Work out the finished part from the listing and answer in its coordinate system (mm). A direction names the side the tool comes from. Give positions to 0.01 mm unless a question says otherwise; leave off trailing zeros. Order: outer loops, then holes, each group sorted by start corner. A loop starts at its lowest first (then second) coordinate and runs counter-clockwise, first axis right, second up.
Autodesk Inventor part; units mm, degrees
ref_plane "YZ Plane" through (0, 0, 0) normal (1, 0, 0) x (0, 1, 0)
ref_plane "XZ Plane" through (0, 0, 0) normal (0, 1, 0) x (-1, 0, 0)
ref_plane "XY Plane" through (0, 0, 0) normal (0, 0, 1) x (1, 0, 0)
sketch "Sketch1" plane through (0, 0, 0) normal (0, 0, 1) x (1, 0, 0)
  line L0 (0, 0) -> (-25.4, 0)
  line L1 (-25.4, 0) -> (-25.4, 25.4)
  line L2 (-25.4, 25.4) -> (0, 25.4)
  line L3 (0, 25.4) -> (0, 0)
  line L4 (-3.175, 22.225) -> (-22.225, 22.225)
  line L5 (-22.225, 22.225) -> (-22.225, 3.175)
  line L6 (-22.225, 3.175) -> (-3.175, 3.175)
  line L7 (-3.175, 3.175) -> (-3.175, 22.225)
  dimension "d2" = 25.4
  dimension "d4" = 25.4
  dimension "d5" = 3.175
extrude "Extrusion1" add sketch "Sketch1" along normal blind 72.39
sketch "Sketch2" plane through (-25.4, 25.4, 0) normal (0, 1, 0) x (1, 0, 0)
  line L0 (0, 0) -> (25.4, 0)
  line L1 (0, 0) -> (0, -72.39)
  line L2 (0, 0) -> (0, -1.905)
  line L3 (12.7, 0) -> (12.7, -1.905)
  line L4 (12.7, -1.905) -> (0, 0)
  line L5 (12.7, -1.905) -> (25.4, 0)
  line L6 (25.4, 0) -> (25.4, -72.39)
  line L7 (12.7, -1.905) -> (8.9322, -27.024)
  line L8 (12.7, -1.905) -> (16.4678, -27.024)
  line L9 (0, -25.6842) -> (8.9322, -27.024)
  line L10 (16.4678, -27.024) -> (25.4, -25.6842)
  line L11 (8.9322, -27.024) -> (17.0812, -28.2463)
  line L12 (16.4678, -27.024) -> (8.6718, -28.1934)
  dimension "d8" = 1.905
  dimension "d9" = 1.905
  dimension "d23" = 25.4
  dimension "d24" = 90
  dimension "d25" = 25.4
  dimension "d26" = 90
extrude "Extrusion2" cut sketch "Sketch2" against normal blind 25.4 contours L4 L7 L9 L1 | L0 L3 L4 | L0 L5 L3 | L5 L6 L10 L8
sketch "Sketch3" plane through (-25.4, 25.4, 72.39) normal (0, 1, 0) x (1, 0, 0)
  line L0 (25.4, 0) -> (0, 0)
  line L1 (25.4, 46.7058) -> (25.4, 0)
  line L2 (12.7, 0) -> (12.7, 70.485) construction
  line L3 (12.7, 0) -> (12.7, 6.35)
  circle A0 centre (12.7, 6.35) radius 3.3782
  circle A1 centre (12.7, 19.05) radius 3.3782
  circle A2 centre (12.7, 31.75) radius 3.3782
  point P0 (25.4, 72.39)
  dimension "d12" = 6.35
  dimension "d13" = 6.7564
  dimension "d16" = 12.7
extrude "Extrusion3" cut sketch "Sketch3" against normal blind 25.4
sketch "Sketch4" plane through (-12.7, 0, 15.24) normal (0, -1, 0) x (1, 0, 0)
  arc A0 (-1.55, -3.0016) -> (1.55, -3.0016) centre (0, 0) ccw
  line L0 (-3.7678, 11.784) -> (0, -13.335)
  line L1 (0, -13.335) -> (3.7678, 11.784)
  point P0 (12.7, -15.24)
extrude "Extrusion4" cut sketch "Sketch4" against normal blind 25.4
sketch "Sketch5" plane through (-25.4, 0, 72.39) normal (0, -1, 0) x (1, 0, 0)
  arc A0 (15.0625, -54.7353) -> (10.3375, -54.7353) centre (12.7, -57.15) ccw
  line L0 (12.7, -70.485) -> (16.4678, -45.366)
  line L1 (8.9322, -45.366) -> (12.7, -70.485)
  circle A1 centre (12.7, -44.45) radius 3.3782
  line L2 (8.9322, -45.366) -> (12.7, -44.45)
  line L3 (12.7, -44.45) -> (16.4678, -45.366)
  point P0 (25.4, -72.39)
extrude "Extrusion5" cut sketch "Sketch5" against normal blind 25.4 contours A0 L1 L2 A1 L3 L0 | A1 L2 L3 picked at (14.5428, -45.7157)
sketch "Sketch8" plane through (-12.7, 25.4, 15.24) normal (0, 1, 0) x (1, 0, 0)
  arc A0 (-2.3625, -2.4147) -> (2.3625, -2.4147) centre (0, 0) ccw
  line L0 (2.3625, -2.4147) -> (1.55, 3.0016)
  arc A1 (1.55, 3.0016) -> (-1.55, 3.0016) centre (0, 0) ccw
  line L1 (-1.55, 3.0016) -> (-2.3625, -2.4147)
  point P0 (12.7, 15.24)
extrude "Extrusion6" cut sketch "Sketch8" against normal blind 25.4
properties part number "V mount" material "Aluminum 6061"
1. The part is cut by section C-C (z = 35.5). Write down the section's boundary in (x, y) (3 decimals), then the cut area to 3 significant figures.
Findings below:
outline: (-25.4, 0) - (0, 0) - (0, 25.4) - (-25.4, 25.4) - close; hole (-22.225, 3.175) - (-3.175, 3.175) - (-3.175, 22.225) - (-22.225, 22.225) - close
area: 282 mm2
2. A straight line is drawn through the part: probe 1 along Y at (x, z) = (-21.75, 45.5) (3 decimals). Find the intervals that lie inside material, in ascending order.
Findings below:
probe 1: y = 0 to 3.175, 22.225 to 25.4
3. The part is cut by section A-A (z = 66.04). Write down the section's boundary in (x, y) (3 decimals), then the cut area to 3 significant figures.
Findings below:
outline: (-25.4, 0) - (-16.078, 0) - (-16.078, 3.175) - (-22.225, 3.175) - (-22.225, 22.225) - (-16.078, 22.225) - (-16.078, 25.4) - (-25.4, 25.4) - close; (-9.322, 0) - (0, 0) - (0, 25.4) - (-9.322, 25.4) - (-9.322, 22.225) - (-3.175, 22.225) - (-3.175, 3.175) - (-9.322, 3.175) - close
area: 239 mm2
4. The part is cut by section D-D (y = 12.75). Write down the section's boundary in (x, z) (3 decimals).
Findings below:
outline: (-25.4, 25.684) - (-22.225, 26.16) - (-22.225, 72.39) - (-25.4, 72.39) - close; (-3.175, 26.16) - (0, 25.684) - (0, 72.39) - (-3.175, 72.39) - close
5. Which of the six approach directions +Z, -Z, +X, -X, +Y, -Y give full straight-line access (tool end or side, diameter ignored) to faces 4 (the face through (-2, 13, 72.39)), 5 (the face through (-22.981, 12.878, 26.047)), 6 (the face through (-22.225, 13, 49))?
Findings below:
face 4: +Z, +X, -X, +Y, -Y
face 5: -Z, +Y, -Y
face 6: +Z, -Z
6. The part is cut by section B-B (y = 23). Write down the section's boundary in (x, z).
Findings below:
outline: (-25.4, 25.68) - (-16.47, 27.02) - (-12.7, 27.94) - (-8.93, 27.02) - (0, 25.68) - (0, 72.39) - (-25.4, 72.39) - close; hole circle Ø6.76 at (-12.7, 40.64); hole circle Ø6.76 at (-12.7, 53.34); hole circle Ø6.76 at (-12.7, 66.04)
7. The mould has two halves that part along Z. Classify faces 1 (the face through (-3.175, 13, 49)), 2 (the face through (-13.43, 1.61, 56.64)), 3 (the face through (-14.61, 23.79, 27.476)): pulls with the +Z half, pulls with the -Z half, needs draft (parallel to the pull), parting line crosses it, or undercut.
Findings below:
face 1: needs draft
face 2: undercut
face 3: pulls with the -Z half
8. Given P1, Ø6, axis at x = -12.7, z = 53.34, coming from the -Y side; P2, Ø4, axis at x = -10, y = 4.5, coming from the -Z side, each flat-ended and moving along its own axis, determine where each tip first touches the part or whether it passes through.
Findings below:
P1: passes through
P2: stops at z = 26.96
